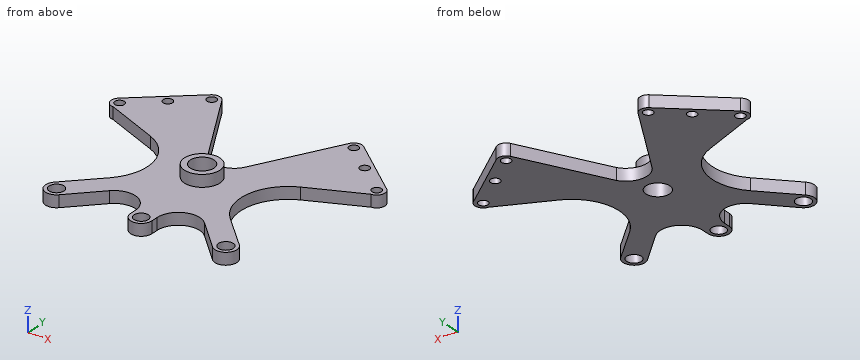
Autodesk Inventor part; units mm, degrees
ref_plane "YZ Plane" through (0, 0, 0) normal (1, 0, 0) x (0, 1, 0)
ref_plane "XZ Plane" through (0, 0, 0) normal (0, 1, 0) x (-1, 0, 0)
ref_plane "XY Plane" through (0, 0, 0) normal (0, 0, 1) x (1, 0, 0)
sketch "Sketch2" plane through (0, 0, 0) normal (0, 0, 1) x (1, 0, 0)
  circle A0 centre (-18.4063, 42.5332) radius 2
  circle A1 centre (-5.7666, 53.1392) radius 2
  circle A2 centre (5.7241, 62.781) radius 2
  circle A3 centre (0, -20) radius 3.1284
  arc A4 (35.5, -17) -> (35.5, -23) centre (35.5, -20) ccw
  circle A5 centre (-18.4063, 42.5332) radius 3.5
  circle A6 centre (5.7241, 62.781) radius 3.5
  line L0 (-18.4063, 42.5332) -> (-5.7666, 53.1392)
  line L1 (-5.7666, 53.1392) -> (5.7241, 62.781)
  line L2 (-20.4063, 45.4055) -> (3.4731, 65.4612)
  line L3 (-15.925, 40.0648) -> (7.9726, 60.0989)
  line L4 (-5.7666, 53.1392) -> (35.5, 15.6275)
  line L5 (-18.5849, 39.0378) -> (4.0074, 29.2589)
  circle A7 centre (0, -20) radius 4.6284
  arc A8 (35.5, -15.5) -> (35.5, -24.5) centre (35.5, -20) ccw
  line L6 (35.5, 15.6275) -> (0, -20)
  line L7 (-3.2742, -16.7286) -> (10.2111, -3.2315)
  line L8 (31, -17.1135) -> (31, -20)
  line L9 (3.2938, -23.2516) -> (15.5951, -10.7907)
  arc A9 (10.2111, -3.2315) -> (4.0074, 29.2589) centre (-3.9371, 10.9045) ccw
  arc A10 (31, -17.1135) -> (15.5951, -10.7907) centre (22, -17.1135) ccw
  line L10 (27.9905, 29.3594) -> (8.7949, 64.4604)
  circle A11 centre (89.4063, 42.5332) radius 2
  circle A12 centre (76.7666, 53.1392) radius 2
  circle A13 centre (65.2759, 62.781) radius 2
  circle A14 centre (71, -20) radius 3.1284
  arc A15 (35.5, -23) -> (35.5, -17) centre (35.5, -20) ccw
  circle A16 centre (89.4063, 42.5332) radius 3.5
  circle A17 centre (65.2759, 62.781) radius 3.5
  line L11 (89.4063, 42.5332) -> (76.7666, 53.1392)
  line L12 (76.7666, 53.1392) -> (65.2759, 62.781)
  line L13 (91.4063, 45.4055) -> (67.5269, 65.4612)
  line L14 (86.925, 40.0648) -> (63.0274, 60.0989)
  line L15 (76.7666, 53.1392) -> (35.5, 15.6275)
  line L16 (89.5849, 39.0378) -> (66.9926, 29.2589)
  circle A18 centre (71, -20) radius 4.6284
  arc A19 (35.5, -24.5) -> (35.5, -15.5) centre (35.5, -20) ccw
  line L17 (35.5, 15.6275) -> (71, -20)
  line L18 (74.2742, -16.7286) -> (60.7889, -3.2315)
  line L19 (40, -17.1135) -> (40, -20)
  line L20 (67.7062, -23.2516) -> (55.4049, -10.7907)
  arc A20 (66.9926, 29.2589) -> (60.7889, -3.2315) centre (74.9371, 10.9045) ccw
  arc A21 (55.4049, -10.7907) -> (40, -17.1135) centre (49, -17.1135) ccw
  line L21 (43.0095, 29.3594) -> (62.2051, 64.4604)
  arc A22 (27.9905, 29.3594) -> (43.0095, 29.3594) centre (35.5, 34.3477) ccw
  line L22 (0, -20) -> (6.5038, -20)
  line L23 (31, -20) -> (35.5, -20)
  line L24 (71, -20) -> (64.4962, -20)
  line L25 (40, -20) -> (35.5, -20)
  circle A23 centre (35.5, 15.6275) radius 5
  point P0 (86, -15)
  point P1 (105.5095, 35.5477)
  point P2 (56.8662, 76.3642)
  point P3 (31, 11.1114)
  point P4 (40, 11.1114)
  dimension "d40" = 7
  dimension "d41" = 7
  dimension "d42" = 11.4907
  dimension "d43" = 16.5
  dimension "d44" = 4
  dimension "d45" = 1.5
  dimension "d46" = 24.1304
  dimension "d47" = 1.5
  dimension "d48" = 1.5
  dimension "d49" = 1.5
  dimension "d51" = 20
  dimension "d52" = 9
  dimension "d54" = 9.2569
  dimension "d55" = 9.0153
  dimension "d56" = 4.5
  dimension "d57" = 0.026
  dimension "d58" = 0.026
  dimension "d59" = 63.405
  dimension "d60" = 5.025
  dimension "d61" = 97.729
  dimension "d62" = 5.369
  dimension "d63" = 5.103
  dimension "d65" = 78.673
  dimension "d66" = 21.327
  dimension "d67" = 94.897
  dimension "d68" = 94.631
  dimension "d69" = 2.271
  dimension "d70" = 94.975
  dimension "d71" = 16.595
  dimension "d72" = 100.026
  dimension "d73" = 0.026
  dimension "d74" = 4.9997
  dimension "d75" = 1.5216
  dimension "d76" = 9.5286
  dimension "d77" = 59.0451
  dimension "d78" = 32.3508
  dimension "d79" = 65.5095
  dimension "d80" = 81.4761
  dimension "d81" = 3.4859
  dimension "d82" = 3.4859
  dimension "d83" = 46.2625
  dimension "d84" = 49.7327
  dimension "d85" = 3.5
  dimension "d86" = 4.9997
  dimension "d87" = 8.5066
  dimension "d88" = 39.9151
  dimension "d89" = 40.9208
  dimension "d90" = 79.1063
  dimension "d91" = 80.2554
  dimension "d92" = 84.8517
  dimension "d93" = 86.0007
  dimension "d94" = 10
extrude "Extrusion1" add sketch "Sketch2" along normal blind 5 contours A5 | A5 L2 A6 L1 A1 L0 | L0 A1 L4 L3 A5 | L3 L4 A23 L6 A7 L7 A9 L5 A5 | A6 | L1 A6 L3 L4 A1 | L3 A6 L10 A22 L21 A17 L14 L15 A23 L4 | L15 L14 A16 L16 A20 L18 A18 L17 A23 | A23 L17 A18 L24 L20 A21 L19 A19 A8 L8 A10 L9 L22 A7 L6 | A7 L6 A3 L22 | L15 A12 L11 A16 L14 | L14 A17 L12 A12 L15 | A7 L22 A3 L6 | A7 L22 L9 | A17 | L17 A14 L24 A18 | A18 L24 A14 L17 | A16 | L13 A16 L11 A12 L12 A17 | A18 L20 L24 | L23 A4 A15 L25 A19 A8 | A8 A19 L25 A15 A4 L23
sketch "Sketch3" plane through (0, 0, 5) normal (0, 0, 1) x (1, 0, 0)
  point P0 (0, 0)
sketch "Sketch4" plane through (0, 0, 5) normal (0, 0, 1) x (1, 0, 0)
  circle A0 centre (35.5, 15.6275) radius 5
  circle A1 centre (35.5, 15.6275) radius 7.5
  point P0 (0, 0)
  dimension "d97" = 15
extrude "Extrusion2" add sketch "Sketch4" along normal blind 5
properties part number "batteryclip2"
CAD build for the part. Positions are in the model's coordinates, mm. Give positions to 0.01 mm unless a question says otherwise; leave off trailing zeros. Loops run counter-clockwise (first coordinate to the right, second up) from the corner with the lowest first, then second, coordinate; pieces in that order, holes last. Notation, with made-up numbers: M 13,-26.5 L 29,-26.5 A13 ccw 29,-16.5 Z; hole C 62.25,2.5 d6. An arc over 180 degrees is marked long. Answer in a Markdown table with one row per item. Add a question column.
Item 1: Band-saw the part on B-B on y = 57.5. Give the cut face in (x, z).
Item 2: Band-saw the part on D-D on y = 33. Give the cut face in (x, z), then the cut area to 3 significant figures.
Item 3: Band-saw the part on A-A on x = 35.5. Give the cut face in (y, z), then the cut area to 3 significant figures.
Item 4: Band-saw the part on C-C on z = 3. Give the number of separate pieces and of enclosed holes in the cut face, then the cut area to 3 significant figures.
Item 5: Probe probe 1 along Y at (x, z) = (35.5, 1.7); probe 2 along Y at (x, z) = (0, 2.75); probe 3 along X at (y, z) = (43.5, 4). List the from-to ranges inside material, lowest first.
Item 6: Drop flat-ended pins along their axis: P1, Ø4, axis at x = 53, y = 14.5, coming from the +Z side; P2, Ø2.5, axis at x = -5.77, y = 53.14, coming from the +Z side; P3, Ø6, axis at y = 48, z = 7, coming from the -X side; P4, Ø1.5, axis at x = 43.5, z = 2.5, coming from the -Y side. Give the stop position or say it passes through.
Reply:
| question | item | result |
|---|---|---|
| 1 | outline | M -6.01,0 L 12.6,0 L 12.6,5 L -6.01,5 Z; M 58.4,0 L 77.01,0 L 77.01,5 L 58.4,5 Z |
| 2 | outline | M -4.64,0 L 26,0 L 26,5 L -4.64,5 Z; M 45,0 L 75.64,0 L 75.64,5 L 45,5 Z |
| 2 | area | 306 mm^2 |
| 3 | outline | M -24.5,0 L -23,0 L -23,5 L -24.5,5 Z; M -17,0 L 10.63,0 L 10.63,10 L 8.13,10 L 8.13,5 L -17,5 Z; M 20.63,0 L 25.33,0 L 25.33,5 L 23.13,5 L 23.13,10 L 20.63,10 Z |
| 3 | area | 194 mm^2 |
| 4 | separate pieces | 1 |
| 4 | enclosed holes | 10 |
| 4 | area | 4,050 mm^2 |
| 5 | probe 1 | y = -24.5 to -23, -17 to 10.63, 20.63 to 25.33 |
| 5 | probe 2 | y = -24.63 to -23.13, -16.87 to -13.45, 30.99 to 62.54 |
| 5 | probe 3 | x = -21.77 to -20.16, -16.66 to 20.26, 50.74 to 87.66, 91.16 to 92.77 |
| 6 | P1 | stops at z = 5 |
| 6 | P2 | passes through |
| 6 | P3 | stops at x = -19.98 |
| 6 | P4 | stops at y = -10.64 |
